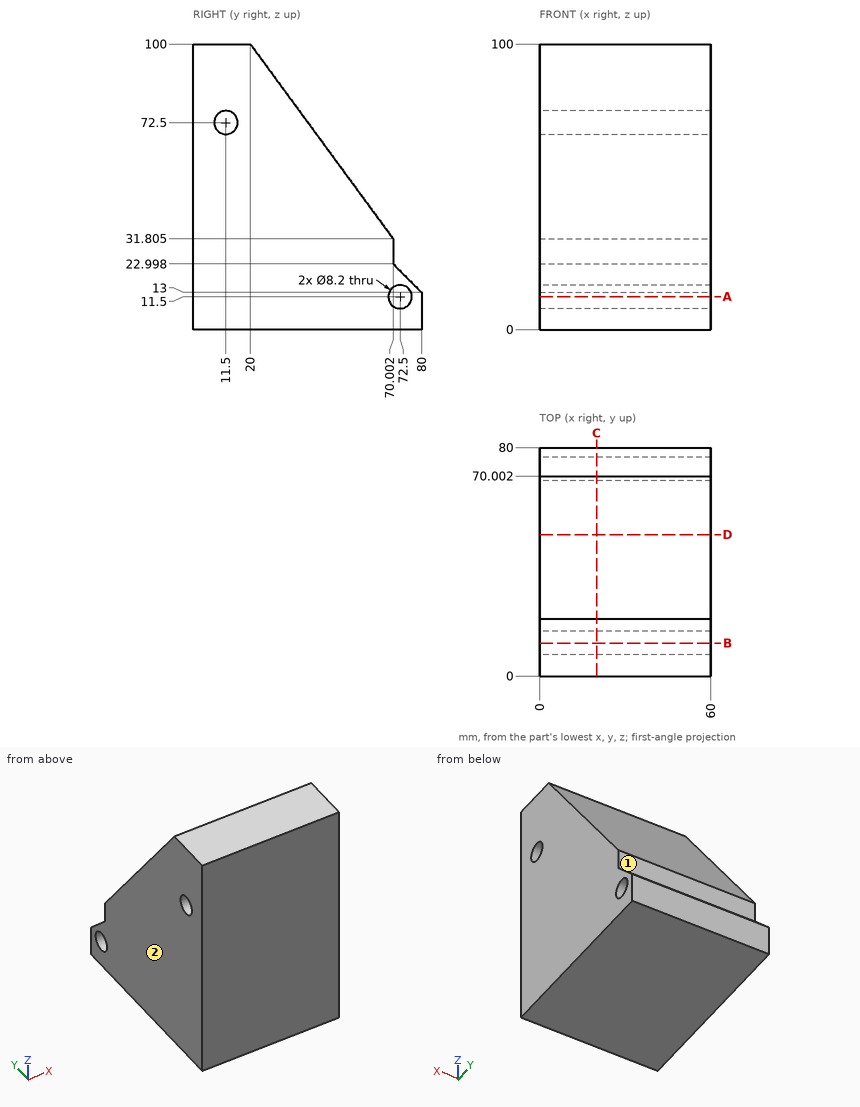
Drawing for the job (mm, zero at the part's lowest x, y, z). A direction names the side the tool comes from. Give positions to 0.01 mm unless a question says otherwise; leave off trailing zeros. Order: outer loops, then holes, each group sorted by start corner. A loop starts at its lowest first (then second) coordinate and runs counter-clockwise, first axis right, second up. Notation, with made-up numbers: M -1.75,-32.75 L 46.25,-32.75 A22 cw 46.25,-0.75 Z; hole C -24.5,41.5 d11. An arc over 180 degrees is marked long. Use a Markdown table: item, result. Add a question column.
(1) Drop flat-ended pins along their axis: P1, Ø7, axis at x = 40.5, z = 29, coming from the +Y side; P2, Ø5, axis at x = 52.5, y = 48.5, coming from the +Z side. Give the stop position or say it passes through.
(2) Saw through at C-C, the plane x = 20. Give the cut face in (y, z) (1 decimal).
(3) Saw through at A-A, the plane z = 11.5. Give the cut face in (x, y).
(4) Saw through at B-B, the plane y = 11.5. Give the cut face in (x, z), and give its area (3 significant figures).
(5) 3-axis set-ups, long thin cutter, end or side, ignore diameter. For the marked faces 1 and 2: which of +Z, -Z, +X, -X, +Y, -Y reach the whole face in a straight line?
(6) Saw through at D-D, the plane y = 49.5. Give the cut face in (x, z), and give its area (3 significant figures).
(7) Probe line 1 along Y through (x, z) = (41.5, 11.5); line 2 along Y through (x, z) = (44, 25); line 3 along Z through (x, y) = (52.5, 69) (1 decimal). List the from-to ranges inside material, lowest first. Write a range as [from, to].
Answer key:
| question | item | result |
|---|---|---|
| 1 | P1 | y = 70 |
| 1 | P2 | z = 64.54 |
| 2 | outline | M 0,0 L 80,0 L 80,13 L 70,23 L 70,31.8 L 20,100 L 0,100 Z; hole C 11.5,72.5 d8.2; hole C 72.5,11.5 d8.2 |
| 3 | outline | M 0,0 L 60,0 L 60,68.4 L 0,68.4 Z; M 0,76.6 L 60,76.6 L 60,80 L 0,80 Z |
| 4 | outline | M 0,0 L 60,0 L 60,68.4 L 0,68.4 Z; M 0,76.6 L 60,76.6 L 60,100 L 0,100 Z |
| 4 | area | 5,510 mm^2 |
| 5 | face 1 | +Z, +X, -X, +Y |
| 5 | face 2 | +Z, -Z, -X, +Y, -Y |
| 6 | outline | M 0,0 L 60,0 L 60,59.77 L 0,59.77 Z |
| 6 | area | 3,590 mm^2 |
| 7 | line 1 | [0, 68.4], [76.6, 80] |
| 7 | line 2 | [0, 70] |
| 7 | line 3 | [0, 9.4], [13.6, 33.2] |
